from build123d import *

# Parameters (mm, degrees)
CUT_EXTRUDE_1_DEPTH = 3.5


with BuildPart() as part:
    # 草图1 → 旋转1 (revolve)
    with BuildSketch(Plane.XY):
        Polygon((-185, 25), (185, 25), (185, 12.5), (205, 12.5), (205, 10), (245, 10), (245, 8.5), (275, 8.5), (275, 0), (235, 0), (-235, 0), (-235, 10), (-205, 10), (-205, 12.5), (-185, 12.5), align=None)
    revolve(axis=Axis((-235, 0, 0), (1, 0, 0)))

    # 草图2 → 切除-拉伸1 (cut)
    with BuildSketch(Plane(origin=(0, 8.5, 0), x_dir=(1, 0, 0), z_dir=(0, 1, 0))):
        with BuildLine():
            Line((250, 3), (270, 3))
            ThreePointArc((270, 3), (273, 0), (270, -3))
            Line((270, -3), (250, -3))
            ThreePointArc((250, -3), (247, 0), (250, 3))
        make_face()
    extrude(amount=-CUT_EXTRUDE_1_DEPTH, mode=Mode.SUBTRACT)


solid = part.part
Part model, mm, in its own coordinate system. A direction names the side the tool comes from. Coordinates: 2 decimals unless noted, no trailing zeros. Loops run counter-clockwise (first coordinate to the right, second up) from the corner with the lowest first, then second, coordinate; pieces in that order, holes last. Notation, with made-up numbers: M 64,13 L 116,13 A24 ccw 116,40 Z; hole C -16,-5 d8. An arc over 180 degrees is marked long. Use a Markdown table: item, result. Add a question column.
Q1. Cut at A-A (y = 0). Write the cut outline in (x, z).
Q2. Which spindle directions (+Z, -Z, +X, -X, +Y, -Y) get a long thin tool onto all of the face, cutting with end or side? Do faces 1 (the cylindrical face through (2.59, 23.846, 7.509)), 2 (the flat face through (245, -4.5, -7.4)), 3 (the cylindrical face through (-194.86, 11.923, 3.755)). Say none if no direction does.
Q3. Probe L1, parallel to X at y = 8.5, z = 9.5; L2, parallel to X at y = -6, z = -9; L3, parallel to Y at x = -204, z = 10. List the from-to ranges inside material, lowest first.
Q4. Cut at B-B (x = 16.5). Write the cut outline in (y, z), and give its area (3 significant figures).
Q5. Pin check, flat tips, straight feed: P1, Ø8, axis at x = -28.5, z = 19, coming from the +Y side; P2, Ø1.5, axis at x = 27, y = -7.5, coming from the +Z side; P3, Ø3, axis at x = 254.5, z = -1, coming from the +Y side. Stop position of each tip, or through.
Q6. Cut at C-C (z = -19). Write the cut outline in (x, y).
Worked out:
| question | item | result |
|---|---|---|
| 1 | outline | M -235,-10 L -205,-10 L -205,-12.5 L -185,-12.5 L -185,-25 L 185,-25 L 185,-12.5 L 205,-12.5 L 205,-10 L 245,-10 L 245,-8.5 L 275,-8.5 L 275,8.5 L 245,8.5 L 245,10 L 205,10 L 205,12.5 L 185,12.5 L 185,25 L -185,25 L -185,12.5 L -205,12.5 L -205,10 L -235,10 Z |
| 2 | face 1 | +X, -X |
| 2 | face 2 | +X |
| 2 | face 3 | -X |
| 3 | L1 | x = -185 to 185 |
| 3 | L2 | x = -205 to 205 |
| 3 | L3 | y = -7.5 to 7.5 |
| 4 | outline | C 0,0 d50 |
| 4 | area | 1,960 mm2 |
| 5 | P1 | stops at y = 20 |
| 5 | P2 | stops at z = 24.07 |
| 5 | P3 | stops at y = 5 |
| 6 | outline | M -185,-16.25 L 185,-16.25 L 185,16.25 L -185,16.25 Z |
